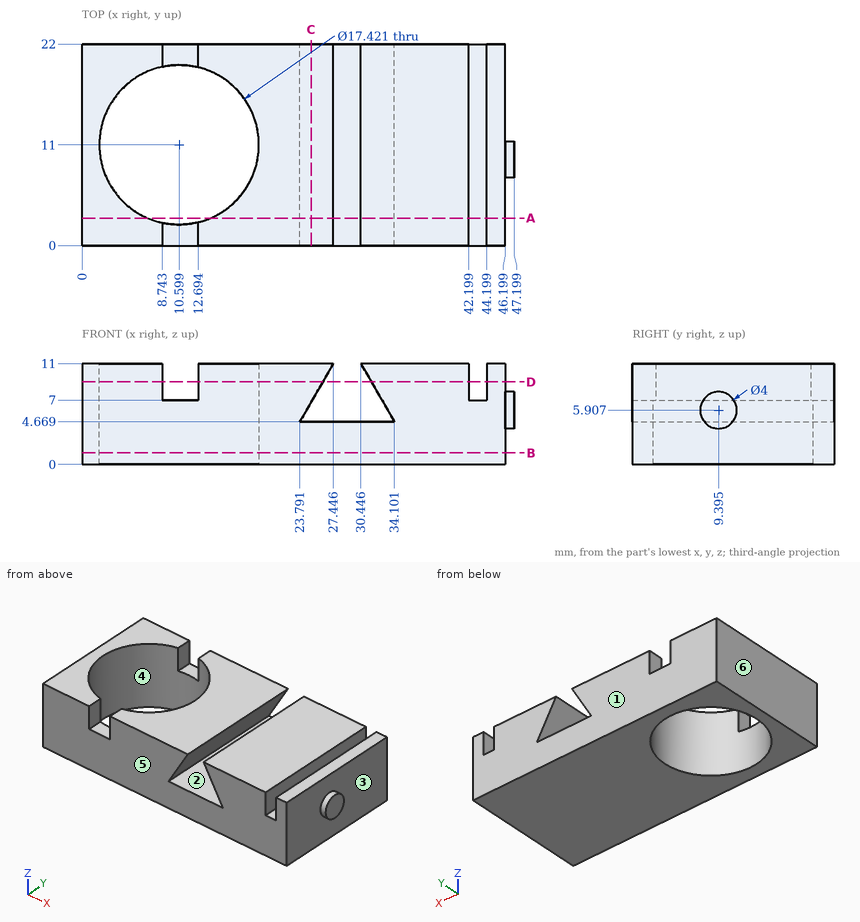
For this review, use the dimensioned drawing (mm, ordinates from the lowest corner) and the shaded views. A direction names the side the tool comes from. Round coordinates to 2 decimals unless told otherwise and drop trailing zeros. Write each loop counter-clockwise with the first axis right and the second up, starting at its lowest first coordinate (ties: lowest second). Pieces come first, ordered by that corner, then holes. Notation, with made-up numbers: (30, 0) -> (75, 0) arc R21 cw to (75, 26) -> close; hole circle Ø3 at (74.25, -28.5). An arc over 180 degrees is marked (long way). Use CSV: the item, a comma, the result in double quotes.
Q1. Consider section B-B (z = 1.25). Give the boundary of the cut face in (x, y).
Checks:
outline,"(0, 0) -> (46.2, 0) -> (46.2, 22) -> (0, 22) -> close; hole circle Ø17.42 at (10.6, 11)"
Q2. Mouldability with a two-part tool opening along X and no side actions: class the marked faces 3, 4, 5 and 6 as released by +X, released by -X, zero draft, split by the parting line, or undercut.
Checks:
face 3,"released by +X"
face 4,"undercut"
face 5,"zero draft"
face 6,"released by -X"
Q3. For the marked faces 1 and 2, list the 3-axis set-ups (+Z, -Z, +X, -X, +Y, -Y) from which the entire face can be reached by the end or side of a thin tool; tool diameter is ignored.
Checks:
face 1,"+Z, -Z, +X, -X, +Y"
face 2,"+Y, -Y"
Q4. To check wall thickness, follow probe 1 along X at (y, z) = (12.5, 7.5) (1 decimal); probe 2 along X at (y, z) = (11, 7.75); probe 3 along X at (y, z) = (11, 5). State the ranges of each line that lie inside material, in increasing order. Write a range as [from, to].
Checks:
probe 1,"[0, 2], [19.2, 25.4], [32.5, 42.2], [44.2, 46.2]"
probe 2,"[0, 1.89], [19.31, 25.57], [32.32, 42.2], [44.2, 46.2]"
probe 3,"[0, 1.89], [19.31, 23.98], [33.91, 47.2]"
Q5. For pin 1 Ø5 at (x, z) = (36, 7.5) entering from -Y; pin 2 Ø1.2 at (y, z) = (8.5, 9) entering from +X; pin 3 Ø1 at (x, y) = (43, 9.5) entering from +Z; pin 4 Ø2 at (x, y) = (5, 15) entering from -Z, all flat-tipped, find the tip position at first contact; note any pin that passes through.
Checks:
pin 1,"y = 0"
pin 2,"x = 46.2"
pin 3,"z = 7"
pin 4,"through"
Q6. Consider section D-D (z = 9). Give the boundary of the cut face in (x, y) (1 decimal).
Checks:
outline,"(0, 0) -> (8.7, 0) -> (8.7, 2.5) arc R8.7 cw to (8.7, 19.5) -> (8.7, 22) -> (0, 22) -> close; (12.7, 0) -> (26.3, 0) -> (26.3, 22) -> (12.7, 22) -> (12.7, 19.5) arc R8.7 cw to (12.7, 2.5) -> close; (31.6, 0) -> (42.2, 0) -> (42.2, 22) -> (31.6, 22) -> close; (44.2, 0) -> (46.2, 0) -> (46.2, 22) -> (44.2, 22) -> close"
Q7. Consider section C-C (x = 25). Give the boundary of the cut face in (y, z), then the cut area to 3 significant figures.
Checks:
outline,"(0, 0) -> (22, 0) -> (22, 4.67) -> (0, 4.67) -> close; (0, 6.76) -> (22, 6.76) -> (22, 11) -> (0, 11) -> close"
area,"196 mm²"
Q8. Consider section A-A (y = 3). Give the boundary of the cut face in (x, z) (1 decimal), then the cut area to 3 significant figures.
Checks:
outline,"(0, 0) -> (7.2, 0) -> (7.2, 11) -> (0, 11) -> close; (14, 0) -> (46.2, 0) -> (46.2, 11) -> (44.2, 11) -> (44.2, 7) -> (42.2, 7) -> (42.2, 11) -> (30.4, 11) -> (34.1, 4.7) -> (23.8, 4.7) -> (27.4, 11) -> (14, 11) -> close"
area,"382 mm²"
